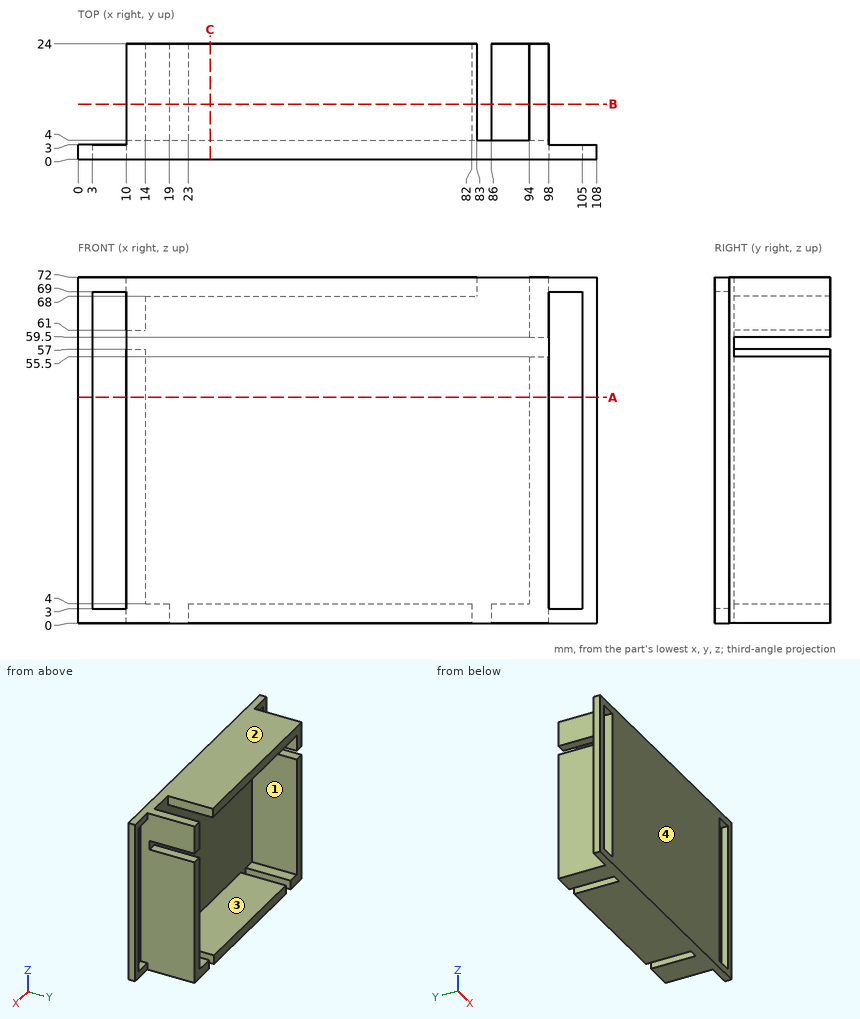
Print and shaded views of the part. All mm, measured from the part's lowest x, y and z. A direction names the side the tool comes from. Give positions to 0.01 mm unless a question says otherwise; leave off trailing zeros. Order: outer loops, then holes, each group sorted by start corner. A loop starts at its lowest first (then second) coordinate and runs counter-clockwise, first axis right, second up. Notation, with made-up numbers: M 60.5,66 L 75.5,66 A21 ccw 75.5,86 Z; hole C -38,34 d3. An arc over 180 degrees is marked long. Use one line per item in the form item = value.
Q1. Slice it at C-C, the plane x = 27.5. Write the cut outline in (y, z), and give its area (3 significant figures).
Conclusion:
outline = M 0,0 L 24,0 L 24,4 L 4,4 L 4,68 L 24,68 L 24,72 L 0,72 Z
area = 448 mm2
Q2. Pin check, flat tips, straight feed: P1, Ø4, axis at x = 91.5, y = 9, coming from the +Z side; P2, Ø6, axis at y = 18.5, z = 18.5, coming from the +X side; P3, Ø4.5, axis at y = 15.5, z = 1, coming from the -X side. Stop position of each tip, or through.
Conclusion:
P1 = 4
P2 = 98
P3 = 10
Q3. Slice it at B-B, the plane y = 11.5. Write the cut outline in (x, z).
Conclusion:
outline = M 10,0 L 19,0 L 19,4 L 14,4 L 14,57 L 10,57 Z; M 10,61 L 14,61 L 14,68 L 83,68 L 83,72 L 10,72 Z; M 23,0 L 82,0 L 82,4 L 23,4 Z; M 86,0 L 98,0 L 98,55.5 L 94,55.5 L 94,4 L 86,4 Z; M 94,59.5 L 98,59.5 L 98,72 L 94,72 Z
Q4. Which spindle directions (+Z, -Z, +X, -X, +Y, -Y) get a long thin tool onto all of the face, cutting with end or side? Do the marked faces 3 and 4. Say none if no direction does.
Conclusion:
face_3 = +Y
face_4 = +Z, -Z, +X, -X, -Y
Q5. Slice it at A-A, the plane z = 47. Write the cut outline in (x, y), and give its area (3 significant figures).
Conclusion:
outline = M 0,0 L 3,0 L 3,3 L 0,3 Z; M 10,0 L 98,0 L 98,24 L 94,24 L 94,4 L 14,4 L 14,24 L 10,24 Z; M 105,0 L 108,0 L 108,3 L 105,3 Z
area = 530 mm2
Q6. Wall check: probe 1 along X at (y, z) = (1.75, 9.5); probe 2 along Z at (x, y) = (64, 20.5); probe 3 along X at (y, z) = (20.5, 14.5). Give the ranges that are in metal, low to high.
Conclusion:
probe_1 = 0 to 3, 10 to 98, 105 to 108
probe_2 = 0 to 4, 68 to 72
probe_3 = 10 to 14, 94 to 98
Q7. Pull direction X, two halves, no side cores. Call the marked faces 1 and 2: released by +X, released by -X, zero draft, split by the parting line, or undercut.
Conclusion:
face_1 = undercut
face_2 = zero draft
